Input: part model. Units: mm. Frame: model coordinates. Coordinates: 2 decimals unless noted, no trailing zeros. Order: outer loops, then holes, each group sorted by start corner. A loop starts at its lowest first (then second) coordinate and runs counter-clockwise, first axis right, second up. Notation, with made-up numbers: (11.5, -5.5) - (55.5, -5.5) arc R20 cw to (55.5, 7.5) - close; hole circle Ø2 at (-10, 17). An arc over 180 degrees is marked (long way). Answer as CSV lines item,"result". Start each with the question number.
Item 1: First-contact query: pin 1 (6 mm diameter, centred on x = -8.5, z = 89, fed in from +Y); pin 2 (1.5 mm diameter, centred on x = -13.5, z = -65, fed in from +Y); pin 3 (3 mm diameter, centred on x = -15, z = -68, fed in from -Y). Flat tips, straight axial feed; report the tip coordinate or a pass-through.
Item 2: Section C-C (x = -18.5). Output: boundary loops of the cut face in (y, z), and give its area (3 significant figures).
Item 3: Section D-D (x = -3.25). Output: boundary loops of the cut face in (y, z).
Item 4: Material intervals for line 1 along Z through (x, y) = (-21.25, 48); line 2 along Z through (x, y) = (-10.75, 95); line 3 along Y through (x, z) = (-5.5, -98), sorted ascending.
from build123d import *

# Parameters (mm, degrees)
F0_W     = 300
F0_H     = 250
F1_DEPTH = 25
F2_SIZE  = 24.99999


# Not quite as in the source:
# - a fillet or chamfer is up to 0.001 mm smaller than in the source, because OpenCascade refuses the exact size


with BuildPart() as f1:
    # F0 (on Right) → F1 (new body)
    with BuildSketch(Plane.YZ):
        Rectangle(F0_W, F0_H)
    extrude(amount=-F1_DEPTH)

    # F2 (size 25 in the source; OpenCascade refuses exactly that, so slightly less here)
    f2_edges = [f1.edges().sort_by_distance(p)[0] for p in [
        (0, 0, 125),
        (0, -150, 0),
        (0, 0, -125),
        (0, 150, 0),
    ]]
    chamfer(f2_edges, length=F2_SIZE)


solid = f1.part
Determined:
1,pin 1,"stops at y = 136.5"
1,pin 2,"stops at y = 139.25"
1,pin 3,"stops at y = -141.5"
2,outline,"(-143.5, -118.5) - (143.5, -118.5) - (143.5, 118.5) - (-143.5, 118.5) - close"
2,area,"68,000 mm^2"
3,outline,"(-128.25, -103.25) - (128.25, -103.25) - (128.25, 103.25) - (-128.25, 103.25) - close"
4,line 1,"z = -121.25 to 121.25"
4,line 2,"z = -110.75 to 110.75"
4,line 3,"y = -130.5 to 130.5"
